from build123d import *

# Parameters (mm, degrees)
BOSS_EXTRUDE1_DEPTH = 1


with BuildPart() as part:
    # Sketch1 → Boss-Extrude1 (new body)
    with BuildSketch(Plane(origin=(0, 60.3, 0), x_dir=(-1, 0, 0), z_dir=(0, 1, 0))):
        Polygon((-1549.465155864, 325.846398989), (-2078.8, 196.077711894), (-2078.8, -196.077711894), (-1549.465155864, -325.846398989), (-1080.847435472, -312.721773603), (-708, -193.60723205), (-708, 193.60723205), (-1080.847435472, 312.721773603), align=None)
        Polygon((-1580, 292.620355358), (-2053.8, 176.466271366), (-2053.8, -176.466271366), (-1580, -292.620355358), align=None, mode=Mode.SUBTRACT)
        Polygon((-1546.790935185, 300.76169876), (-1555, 298.749211626), (-1555, -298.749211626), (-1548.049652364, -300.796951783), (-1085.08461283, -287.83064162), (-1075, -284.608884087), (-1075, 284.608884087), (-1085.08461283, 287.83064162), align=None, mode=Mode.SUBTRACT)
        Polygon((-733, 175.349253107), (-733, -175.349253107), (-1050, -276.622068957), (-1050, 276.622068957), align=None, mode=Mode.SUBTRACT)
    extrude(amount=BOSS_EXTRUDE1_DEPTH)


solid = part.part
The listing builds one solid part. Answer for the finished solid, in the listing's coordinates (mm). A direction names the side the tool comes from. Coordinates: 2 decimals unless noted, no trailing zeros. Loops run counter-clockwise (first coordinate to the right, second up) from the corner with the lowest first, then second, coordinate; pieces in that order, holes last. Notation, with made-up numbers: (81, -15) -> (118, -15) arc R5 cw to (118, -10) -> close; hole circle Ø11 at (57, 86). An arc over 180 degrees is marked (long way). Answer in a Markdown table with one row per item. Add a question column.
1. Consider line 1 (X direction, y = 60.6, z = -129.5); line 2 (Z direction, x = 810.5, y = 61.1); line 3 (Z direction, x = 1840, y = 60.75). Determine where each line is inside the solid, lowest interval first. Write a range as [from, to].
2. The part is cut by section D-D, the plane z = 260.5. Write down the section's boundary in (x, y), then the cut area to 3 significant figures.
3. For faces 1 (the flat face through (1820.22, 60.79, -233.73)), 2 (the flat face through (1810.43, 60.79, 261.87)), determine the directions among +Z, -Z, +X, -X, +Y, -Y from which every point of the face is accessible in a straight line to the end or side of a thin tool.
4. The part is cut by section C-C, the plane x = 1176. Write down the section's boundary in (y, z), then the cut area to 3 significant figures.
5. Determine the mould class of faces 3 (the flat face through (1600, 61.3, -288)), 4 (the flat face through (893.719, 60.793, 226.695)), 5 (the flat face through (897.034, 60.793, -253.998)) for opening direction X: +X half, -X half, draft (parallel to the pull), parting line (faces both ways), or undercut.
6. The part is cut by section B-B, the plane y = 60.95. Write down the section's boundary in (x, z), then the cut area to 3 significant figures.
7. The part is cut by section A-A, the plane z = 114. Write down the section's boundary in (x, y).
Answer below:
| question | item | result |
|---|---|---|
| 1 | line 1 | [708, 733], [1050, 1075], [1555, 1580], [2053.8, 2078.8] |
| 1 | line 2 | [-226.35, -200.11], [200.11, 226.35] |
| 1 | line 3 | [-254.62, -228.88], [228.88, 254.62] |
| 2 | outline | (917.38, 60.3) -> (999.54, 60.3) -> (999.54, 61.3) -> (917.38, 61.3) -> close; (1050, 60.3) -> (1075, 60.3) -> (1075, 61.3) -> (1050, 61.3) -> close; (1555, 60.3) -> (1580, 60.3) -> (1580, 61.3) -> (1555, 61.3) -> close; (1711.02, 60.3) -> (1816.02, 60.3) -> (1816.02, 61.3) -> (1711.02, 61.3) -> close |
| 2 | area | 237 mm2 |
| 3 | face 1 | +Y, -Y |
| 3 | face 2 | +Z, +X, +Y, -Y |
| 4 | outline | (60.3, -315.39) -> (61.3, -315.39) -> (61.3, -290.38) -> (60.3, -290.38) -> close; (60.3, 290.38) -> (61.3, 290.38) -> (61.3, 315.39) -> (60.3, 315.39) -> close |
| 4 | area | 50.0 mm2 |
| 5 | face 3 | draft |
| 5 | face 4 | undercut |
| 5 | face 5 | -X half |
| 6 | outline | (708, -193.61) -> (1080.85, -312.72) -> (1549.47, -325.85) -> (2078.8, -196.08) -> (2078.8, 196.08) -> (1549.47, 325.85) -> (1080.85, 312.72) -> (708, 193.61) -> close; hole (733, -175.35) -> (1050, -276.62) -> (1050, 276.62) -> (733, 175.35) -> close; hole (1075, -284.61) -> (1085.08, -287.83) -> (1548.05, -300.8) -> (1555, -298.75) -> (1555, 298.75) -> (1546.79, 300.76) -> (1085.08, 287.83) -> (1075, 284.61) -> close; hole (1580, -292.62) -> (2053.8, -176.47) -> (2053.8, 176.47) -> (1580, 292.62) -> close |
| 6 | area | 116,000 mm2 |
| 7 | outline | (708, 60.3) -> (733, 60.3) -> (733, 61.3) -> (708, 61.3) -> close; (1050, 60.3) -> (1075, 60.3) -> (1075, 61.3) -> (1050, 61.3) -> close; (1555, 60.3) -> (1580, 60.3) -> (1580, 61.3) -> (1555, 61.3) -> close; (2053.8, 60.3) -> (2078.8, 60.3) -> (2078.8, 61.3) -> (2053.8, 61.3) -> close |
